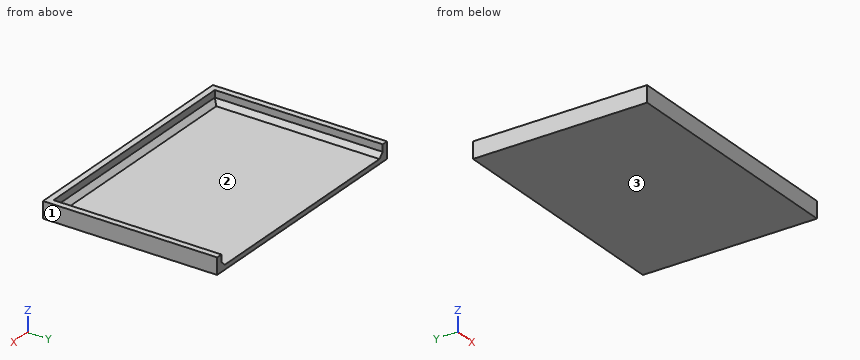
from build123d import *

# Parameters (mm, degrees)
F1_DEPTH = 4.2
F0_W     = 60
F0_H     = 43
F2_DEPTH = 1.2
F3_SIZE  = 1.2


with BuildPart() as f1:
    # F0 (on Top) → F1 (new body)
    with BuildSketch(Plane.XY):
        Polygon((-28.6880440414, 27.4013292328), (-30.2880440414, 27.4013292328), (-30.2880440414, -17.1986707672), (32.9119559586, -17.1986707672), (32.9119559586, 27.4013292328), (31.3119559586, 27.4013292328), (31.3119559586, -15.5986707672), (-28.6880440414, -15.5986707672), align=None)
    extrude(amount=F1_DEPTH)

    # F0 (on Top) → F2 (join)
    with BuildSketch(Plane.XY):
        Polygon((-28.6880440414, 27.4013292328), (-30.2880440414, 27.4013292328), (-30.2880440414, -17.1986707672), (32.9119559586, -17.1986707672), (32.9119559586, 27.4013292328), (31.3119559586, 27.4013292328), (31.3119559586, -15.5986707672), (-28.6880440414, -15.5986707672), align=None)
        with Locations((1.3119559586, 5.9013292328)):
            Rectangle(F0_W, F0_H)
    extrude(amount=F2_DEPTH)

    # F3
    f3_edges = [f1.edges().sort_by_distance(p)[0] for p in [
        (-28.688044, 5.901329, 1.2),
        (1.311956, -15.598671, 1.2),
        (31.311956, 5.901329, 1.2),
    ]]
    chamfer(f3_edges, length=F3_SIZE)


solid = f1.part
Verification items for the finished model (mm, model axes). Face numbers are marked on the shaded views. Coordinates: 2 decimals unless noted, no trailing zeros. Write each loop counter-clockwise with the first axis right and the second up, starting at its lowest first coordinate (ties: lowest second). Pieces come first, ordered by that corner, then holes. Notation, with made-up numbers: M 66,-29 L 119,-29 A25 cw 119,-15 Z; hole C -24.5,81.5 d3. An arc over 180 degrees is marked long. One line per question, with ' | ' between items.
1) Release check for a two-part mould opening along X. For the marked faces 1, 2 and 3 record: +X half, -X half, draft (parallel to the pull), parting line (faces both ways), or undercut.
Solutions:
face 1: +X half | face 2: undercut | face 3: draft
2) Depth check by flat-ended pin: pin 1 Ø8 at (x, y) = (-17, -8) entering from -Z; pin 2 Ø1.4 at (x, z) = (-10.5, 3.5) entering from +Y; pin 3 Ø1.5 at (x, y) = (11.5, 21) entering from +Z. Enter the tip coordinate at first touch or a pass-through.
Solutions:
pin 1: z = 0 | pin 2: y = -15.6 | pin 3: z = 1.2
3) Material ranges on L1, parallel to X at y = -8, z = 3.35; L2, parallel to Z at x = -19.5, y = 9.5; L3, parallel to Y at x = 27, z = 3.75, recorded low to high.
Solutions:
L1: -30.29 to -28.69, 31.31 to 32.91 | L2: 0 to 1.2 | L3: -17.2 to -15.6
4) Sectioned sample at B-B on x = 13. Record the cut outline in (y, z), then the cut area to 3 significant figures.
Solutions:
outline: M -17.2,0 L 27.4,0 L 27.4,1.2 L -14.4,1.2 L -15.6,2.4 L -15.6,4.2 L -17.2,4.2 Z | area: 59.0 mm^2
5) Sectioned sample at A-A on y = 23. Record the cut outline in (x, z), then the cut area to 3 significant figures.
Solutions:
outline: M -30.29,0 L 32.91,0 L 32.91,4.2 L 31.31,4.2 L 31.31,2.4 L 30.11,1.2 L -27.49,1.2 L -28.69,2.4 L -28.69,4.2 L -30.29,4.2 Z | area: 86.9 mm^2
